from build123d import *

# Parameters (mm, degrees)
SKETCH048_W         = 28
SKETCH048_H         = 18
PAD032_DEPTH        = 3
SKETCH049_R         = 7.075
POCKET009_DEPTH     = 18.001
PAD033_START        = -2
PAD033_DEPTH        = 14
SKETCH051_W         = 1.925
SKETCH051_H         = 5
PAD034_DEPTH        = 6
SKETCH052_W         = 5
SKETCH052_H         = 6
PAD035_DEPTH        = 5
SKETCH053_W         = 5
SKETCH053_H         = 6
PAD036_DEPTH        = 5
HOLE004_D           = 2.6
HOLE004_DEPTH       = 25
HOLE004_CBORE_D     = 4
HOLE004_CBORE_DEPTH = 1
SKETCH056_R         = 1.45
POCKET010_DEPTH     = 4
FILLET013_R         = 1
FILLET014_R         = 1


with BuildPart() as part:
    # Sketch048 (on Face1 of CopyPad022) → Pad032 (new body)
    with BuildSketch(Plane(origin=(0, 0, -2), x_dir=(1, 0, 0), z_dir=(0, 0, -1))):
        with Locations((-18.5, 29.3848)):
            Rectangle(SKETCH048_W, SKETCH048_H)
    extrude(amount=PAD032_DEPTH)

    # Sketch049 (on Face2 of Pad032) → Pocket009 (cut, through all)
    with BuildSketch(Plane(origin=(0, -20.3848, -2), x_dir=(-1, 0, 0), z_dir=(0, 1, 0))):
        with Locations((18.5, -9.075)):
            Circle(SKETCH049_R)
    extrude(amount=-POCKET009_DEPTH, mode=Mode.SUBTRACT)

    # Sketch050 (on Face2 of Pocket009) → Pad033 (join)
    with BuildSketch(Plane(origin=(0, -38.3848, -2), x_dir=(1, 0, 0), z_dir=(0, -1, 0)).offset(PAD033_START)):
        with BuildLine():
            ThreePointArc((-11.425, -9.075), (-18.5, -2), (-25.575, -9.075))
            Line((-27.5, -9.075), (-25.575, -9.075))
            ThreePointArc((-9.5, -9.075), (-18.5, -0.075), (-27.5, -9.075))
            Line((-11.425, -9.075), (-9.5, -9.075))
        make_face()
    extrude(amount=-PAD033_DEPTH)

    # Sketch051 (on Face14 of Pad033) → Pad034 (join)
    with BuildSketch(Plane(origin=(0, 0, -11.075), x_dir=(1, 0, 0), z_dir=(0, 0, -1))):
        with Locations((-26.5375, 29.3848)):
            Rectangle(SKETCH051_W, SKETCH051_H)
        with Locations((-10.4625, 29.3848)):
            Rectangle(SKETCH051_W, SKETCH051_H)
    extrude(amount=-PAD034_DEPTH)

    # Sketch052 (on Face18 of Pad034) → Pad035 (join)
    with BuildSketch(Plane(origin=(-27.5, 0, -2), x_dir=(0, -1, 0), z_dir=(-1, 0, 0))):
        with Locations((29.3848, -6.075)):
            Rectangle(SKETCH052_W, SKETCH052_H)
    extrude(amount=PAD035_DEPTH)

    # Sketch053 (on Face17 of Pad035) → Pad036 (join)
    with BuildSketch(Plane(origin=(-9.5, 0, -2), x_dir=(0, 1, 0), z_dir=(1, 0, 0))):
        with Locations((-29.3848, -6.075)):
            Rectangle(SKETCH053_W, SKETCH053_H)
    extrude(amount=PAD036_DEPTH)

    # Hole004
    with Locations(Plane(origin=(0, 0, -5), x_dir=(1, 0, 0), z_dir=(0, 0, -1))):
        with Locations((-7.5, 34.8848), (-29.5, 34.8848), (-29.5, 23.8848), (-7.5, 23.8848)):
            CounterBoreHole(HOLE004_D / 2, HOLE004_CBORE_D / 2, HOLE004_CBORE_DEPTH, depth=HOLE004_DEPTH)

    # Sketch056 → Pocket010 (cut)
    with BuildSketch(Plane(origin=(0, 0, -11.075), x_dir=(1, 0, 0), z_dir=(0, 0, -1))):
        with Locations((-8, 29.3848)):
            Circle(SKETCH056_R)
        with Locations((-29, 29.3848)):
            Circle(SKETCH056_R)
    extrude(amount=-POCKET010_DEPTH, mode=Mode.SUBTRACT)

    # Fillet013
    fillet013_edges = [part.edges().sort_by_distance(p)[0] for p in [
        (-32.5, -31.8848, -8.075),
        (-32.5, -26.8848, -8.075),
    ]]
    fillet(fillet013_edges, radius=FILLET013_R)

    # Fillet014
    fillet014_edges = [part.edges().sort_by_distance(p)[0] for p in [
        (-4.5, -26.8848, -8.075),
        (-4.5, -31.8848, -8.075),
    ]]
    fillet(fillet014_edges, radius=FILLET014_R)


with BuildPart() as part_1:
    # Body006 placement: moved
    add(part.part.moved(Location((1, 32.65, 0))))


solid = part_1.part
Build history of the part. All positions in model axes, mm. A direction names the side the tool comes from. Coordinates: 2 decimals unless noted, no trailing zeros. Order: outer loops, then holes, each group sorted by start corner. A loop starts at its lowest first (then second) coordinate and runs counter-clockwise, first axis right, second up. Notation, with made-up numbers: (38, -18.5) - (66, -18.5) arc R18 ccw to (66, 14.5) - close; hole circle Ø3 at (17.5, 7). An arc over 180 degrees is marked (long way). Write each question's results on one line, items separated by ' | '. Start each with the question number.
Item 1: Flat gauge pins, fed straight in: pin 1 (3 mm diameter, centred on x = -28, z = -7.5, fed in from -Y); pin 2 (2 mm diameter, centred on x = -28, y = -1.5, fed in from -Z); pin 3 (0.9 mm diameter, centred on x = -6.5, y = 3.5, fed in from -Z) (3 decimals). Where does each tip first touch, or does it go through?
Item 2: Tool access for faces 5 (the face through (-7, 0.765, -8)), 6 (the face through (-28, 5.765, -8)), 7 (the face through (-27.2, -2.3, -3)), 8 (the face through (-8.09, -1.02, -4.51)): list every direction of +Z, -Z, +X, -X, +Y, -Y with a clear straight run to the whole face (end or side of a thin tool).
Item 3: Mould opens along X. For faces 1 (the face through (-31.5, 3, -8)), 2 (the face through (-26.592, -2.836, -4.507)), 3 (the face through (-28, 3, -7.075)), 4 (the face through (-3.785, 5.464, -8.033)) say: released by +X, released by -X, zero draft, split by the parting line, or undercut.
Item 4: Band-saw the part on D-D on z = -3.25. Write the cut outline in (x, y), and give its area (3 significant figures).
Item 5: Band-saw the part on B-B on z = -6.75. Write the cut outline in (x, y).
Item 6: Band-saw the part on A-A on x = -6. Write the cut outline in (y, z) (3 decimals), and give its area (3 significant figures).
Item 7: Wall check: probe 1 along Y at (x, z) = (-28.5, -3.3); probe 2 along Y at (x, z) = (-6.5, -4.3); probe 3 along Y at (x, z) = (-28, -8.8). Give the ranges that are in metal, low to high. Write a range as [from, to].
Item 8: Band-saw the part on C-C on x = -9.5. Write the cut outline in (y, z) (3 decimals).
Numbers:
1) pin 1: y = 0.77 | pin 2: z = -4 | pin 3: z = -7.075
2) face 5: +X, -Y | face 6: -X, +Y | face 7: +Z, -Z | face 8: -Z
3) face 1: released by -X | face 2: undercut | face 3: undercut | face 4: released by +X
4) outline: (-31.5, -5.73) - (-3.5, -5.73) - (-3.5, 12.27) - (-31.5, 12.27) - close; hole circle Ø2.6 at (-28.5, -2.23); hole circle Ø2.6 at (-28.5, 8.77); hole circle Ø2.6 at (-6.5, -2.23); hole circle Ø2.6 at (-6.5, 8.77) | area: 483 mm^2
5) outline: (-31.5, 1.77) arc R1 ccw to (-30.5, 0.77) - (-25.39, 0.77) - (-25.39, -3.73) - (-23.1, -3.73) - (-23.1, 10.27) - (-25.39, 10.27) - (-25.39, 5.77) - (-30.5, 5.77) arc R1 ccw to (-31.5, 4.77) - close; (-11.9, -3.73) - (-9.61, -3.73) - (-9.61, 0.77) - (-4.5, 0.77) arc R1 ccw to (-3.5, 1.77) - (-3.5, 4.77) arc R1 ccw to (-4.5, 5.77) - (-9.61, 5.77) - (-9.61, 10.27) - (-11.9, 10.27) - close
6) outline: (-5.735, -5) - (-4.171, -5) - (-4.171, -4) - (-3.435, -4) - (-3.435, -2) - (-5.735, -2) - close; (-1.035, -4) - (-0.298, -4) - (-0.298, -5) - (6.829, -5) - (6.829, -4) - (7.565, -4) - (7.565, -2) - (-1.035, -2) - close; (0.765, -11.075) - (2.215, -11.075) - (2.215, -7.075) - (4.315, -7.075) - (4.315, -11.075) - (5.765, -11.075) - (5.765, -5.075) - (0.765, -5.075) - close; (9.965, -4) - (10.702, -4) - (10.702, -5) - (12.265, -5) - (12.265, -2) - (9.965, -2) - close | area: 58.3 mm^2
7) probe 1: [-5.73, -3.53], [-0.93, 7.47], [10.07, 12.27] | probe 2: [-5.73, -4.23], [-0.23, 6.77], [10.77, 12.27] | probe 3: [0.77, 1.82], [4.72, 5.77]
8) outline: (-5.735, -5) - (12.265, -5) - (12.265, -2) - (-5.735, -2) - close; (-3.735, -11.075) - (10.265, -11.075) - (10.265, -6.952) - (5.765, -6.952) - (5.765, -5.075) - (0.765, -5.075) - (0.765, -6.952) - (-3.735, -6.952) - close
